Design review of the part built by this model. Coordinates are the model's own, in mm. Face numbers are marked on the shaded views. A direction names the side the tool comes from. Give positions to 0.01 mm unless a question says otherwise; leave off trailing zeros. Loops run counter-clockwise (first coordinate to the right, second up) from the corner with the lowest first, then second, coordinate; pieces in that order, holes last. Notation, with made-up numbers: (4, 14) -> (12, 14) arc R13 ccw to (12, 38) -> close; hole circle Ø11 at (57.25, -19.5). An arc over 180 degrees is marked (long way). Use CSV: the item, a comma, the result in double quotes. Start each with the question number.
Item 1: Wall thickness on line 1 along X through (y, z) = (6.25, 0); line 2 along X through (y, z) = (12.4, 0); line 3 along Y through (x, z) = (-2.5, 4.25): over which ranges is each line inside the solid? List them lowest first. Write a range as from..to.
Item 2: Clearance check with flat-ended pins moving along their axes: pin 1 (3 mm diameter, centred on x = 9.5, y = 2, fed in from +Z); pin 2 (3 mm diameter, centred on y = 10, z = 8.5, fed in from -X); pin 3 (3 mm diameter, centred on x = -5.5, y = 11.5, fed in from -Z); pin 4 (12.5 mm diameter, centred on x = 0, z = 0, fed in from -Y). State where each tip first meets the part, or that it passes through.
Item 3: The part is to be moulded in two halves that separate along X. For the marked faces 1, 2 and 3, say which applies: +X half, -X half, draft (parallel to the pull), parting line (faces both ways), or undercut.
Item 4: We need section A-A (z = 0). State the section outline as (x, y) points, plus the area to 3 significant figures.
Item 5: We need section B-B (y = 7). State the section outline as (x, z) points.
Item 6: For the marked faces 4 and 5, list the 3-axis set-ups (+Z, -Z, +X, -X, +Y, -Y) from which the entire face can be reached by the end or side of a thin tool; tool diameter is ignored.
from build123d import *

# Parameters (mm, degrees)
BOSS_EXTRUDE1_DEPTH = 15
CUT_EXTRUDE2_REACH  = 26.281
SKETCH5_R           = 3.5
SKETCH8_R           = 7.75
CUT_EXTRUDE3_DEPTH  = 10


with BuildPart() as part:
    # Sketch2 → Boss-Extrude1 (new body)
    with BuildSketch(Plane(origin=(0, 0, 0), x_dir=(1, 0, 0), z_dir=(0, 1, 0))):
        Polygon((0, 14.43375673), (-12.5, 7.216878365), (-12.5, -7.216878365), (0, -14.43375673), (12.5, -7.216878365), (12.5, 7.216878365), align=None)
    extrude(amount=BOSS_EXTRUDE1_DEPTH)

    # Sketch3 → Cut-Revolve1 (revolve, cut)
    with BuildSketch(Plane(origin=(0, 0, 0), x_dir=(0, 0, -1), z_dir=(1, 0, 0))):
        Polygon((14.43375673, 15), (12.43375673, 15), (14.43375673, 13), align=None)
    cut_revolve1 = revolve(axis=Axis((0, 0, 0), (0, 1, 0)), mode=Mode.SUBTRACT)

    # Mirror1: Cut-Revolve1 across plane
    add(cut_revolve1.mirror(Plane.ZX.offset(7.5)), mode=Mode.SUBTRACT)

    # Sketch5 → Cut-Extrude2 (cut, up to next)
    with BuildSketch(Plane.XZ, mode=Mode.PRIVATE) as cut_extrude2_sk1:
        with Locations(Location((0, 0, 0), (0, 0, 270))):
            Circle(SKETCH5_R)
    cut_extrude2_tool1 = extrude(cut_extrude2_sk1.sketch, amount=-CUT_EXTRUDE2_REACH, mode=Mode.PRIVATE) & part.part
    add(cut_extrude2_tool1.solids().sort_by_distance((0, 0, 0))[0], mode=Mode.SUBTRACT)

    # Sketch8 → Cut-Extrude3 (cut)
    with BuildSketch(Plane.XZ):
        with Locations(Location((0, 0, 0), (0, 0, 270))):
            Circle(SKETCH8_R)
    extrude(amount=-CUT_EXTRUDE3_DEPTH, mode=Mode.SUBTRACT)


solid = part.part
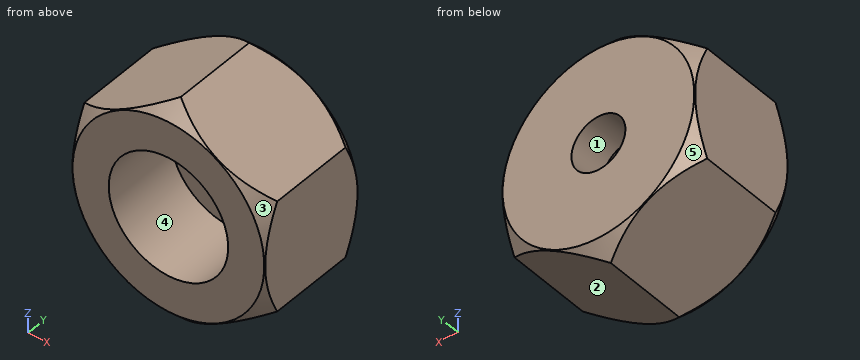
Results found:
1,line 1,"-12.5..-7.75, 7.75..12.5"
1,line 2,"-12.5..-3.5, 3.5..12.5"
1,line 3,"10..15"
2,pin 1,"z = 9.81"
2,pin 2,"x = -12.5"
2,pin 3,"z = -12.12"
2,pin 4,"y = 10"
3,face 1,"undercut"
3,face 2,"+X half"
3,face 3,"parting line"
4,outline,"(-12.5, 0.07) -> (-12.43, 0) -> (-7.75, 0) -> (-7.75, 10) -> (-3.5, 10) -> (-3.5, 15) -> (-12.43, 15) -> (-12.5, 14.93) -> close; (3.5, 10) -> (7.75, 10) -> (7.75, 0) -> (12.43, 0) -> (12.5, 0.07) -> (12.5, 14.93) -> (12.43, 15) -> (3.5, 15) -> close"
4,area,"185 mm²"
5,outline,"(-12.5, -7.22) -> (0, -14.43) -> (12.5, -7.22) -> (12.5, 7.22) -> (0, 14.43) -> (-12.5, 7.22) -> close; hole circle Ø15.5 at (0, 0)"
6,face 4,"-Y"
6,face 5,"+Y"
